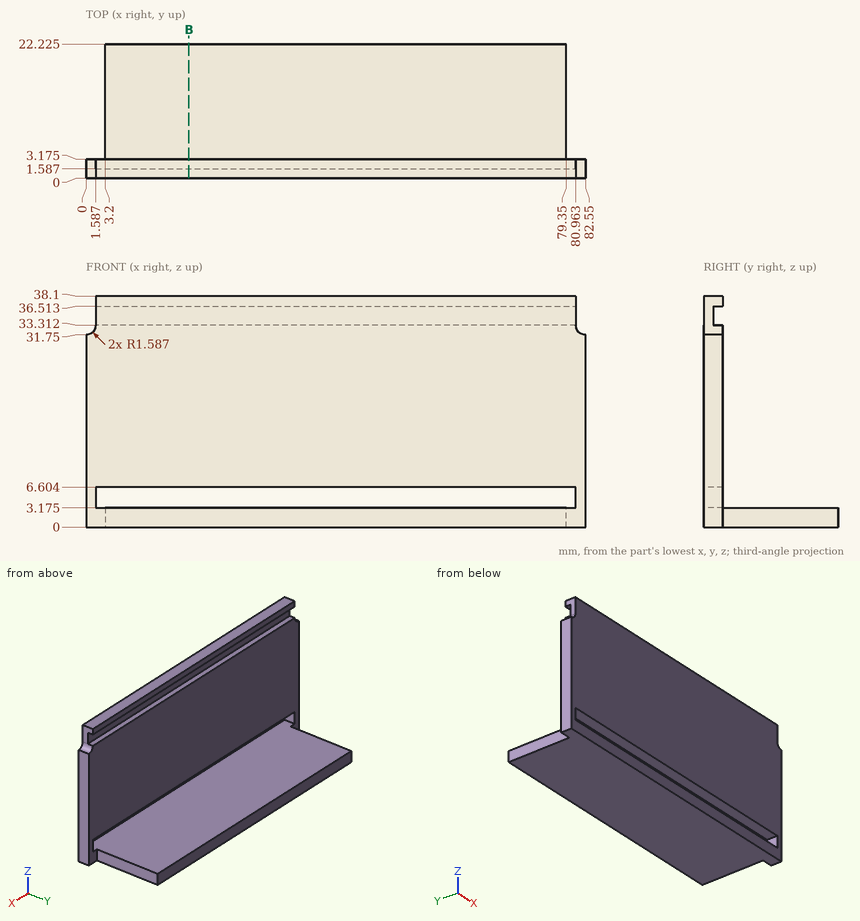
The figure shows three views and two pictorial views of one solid part (mm, origin at its lowest corner). Answer the questions. Coordinates: 2 decimals unless noted, no trailing zeros. Write each loop counter-clockwise with the first axis right and the second up, starting at its lowest first coordinate (ties: lowest second). Pieces come first, ordered by that corner, then holes.
1. Consider line 1 along Z through (x, y) = (42.5, 3) (1 decimal); line 2 along Z through (x, y) = (5.5, 19.25) (1 decimal). Determine where each line is inside the solid, lowest interval first.
Results list:
line 1: z = 0 to 3.2, 6.6 to 33.3, 36.5 to 38.1
line 2: z = 0 to 3.2
2. Flat-ended cylindrical pins translate along their axes: pin 1 (1 mm diameter, centred on y = 1.5, z = 36, fed in from +X); pin 2 (3.5 mm diameter, centred on y = 1, z = 36.5, fed in from -X); pin 3 (4 mm diameter, centred on x = 63, y = 10.5, fed in from +Z) (1 decimal); pin 4 (4 mm diameter, centred on x = 15, z = 10.5, fed in from -Y). Find the tip coordinate at first contact, or state that the pin passes through.
Results list:
pin 1: stops at x = 80.96
pin 2: stops at x = 1.59
pin 3: stops at z = 3.2
pin 4: stops at y = 0
3. The part is cut by section B-B, the plane x = 17. Write down the section's boundary in (y, z) (1 decimal).
Results list:
outline: (0, 0) - (22.2, 0) - (22.2, 3.2) - (0, 3.2) - close; (0, 6.6) - (3.2, 6.6) - (3.2, 33.3) - (1.6, 33.3) - (1.6, 36.5) - (3.2, 36.5) - (3.2, 38.1) - (0, 38.1) - close
